from build123d import *

# Parameters (mm, degrees)
SKETCH1_R           = 2.75
BOSS_EXTRUDE1_DEPTH = 2


with BuildPart() as part:
    # Sketch1 → Boss-Extrude1 (new body)
    with BuildSketch(Plane(origin=(0, 0, 0), x_dir=(0, 0, -1), z_dir=(1, 0, 0))):
        with BuildLine():
            Line((4, 4), (44, 4))
            Line((44, 4), (44, -21))
            ThreePointArc((44, -21), (48, -25), (52, -21))
            Line((52, -21), (52, 4))
            Line((52, 4), (77, 4))
            ThreePointArc((77, 4), (81, 8), (77, 12))
            Line((77, 12), (4, 12))
            ThreePointArc((4, 12), (0, 8), (4, 4))
        make_face()
        with Locations((4, 8)):
            Circle(SKETCH1_R, mode=Mode.SUBTRACT)
        with Locations((77, 8)):
            Circle(SKETCH1_R, mode=Mode.SUBTRACT)
        with Locations((48, -21)):
            Circle(SKETCH1_R, mode=Mode.SUBTRACT)
    extrude(amount=-BOSS_EXTRUDE1_DEPTH)


solid = part.part
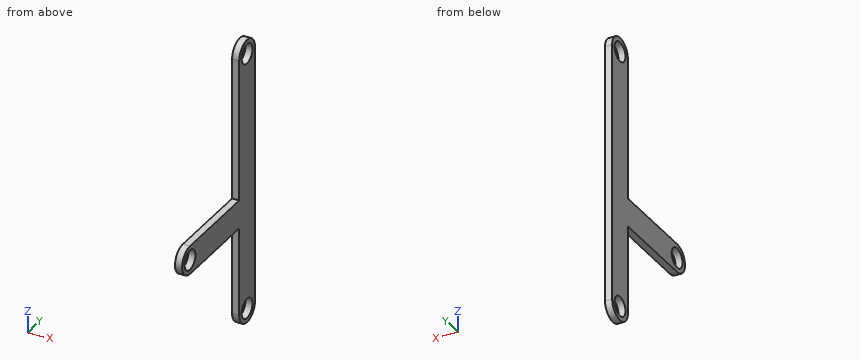
Can you work these out from the model? Positions are in its coordinate system, mm. Give positions to 0.01 mm unless a question says otherwise; leave off trailing zeros. Order: outer loops, then holes, each group sorted by start corner. A loop starts at its lowest first (then second) coordinate and runs counter-clockwise, first axis right, second up. Notation, with made-up numbers: M 39.25,-15 L 65.25,-15 A14 ccw 65.25,7 Z; hole C 4,74.25 d8. An arc over 180 degrees is marked long. Use one line per item in the form item = value. Start each with the question number.
Item 1: Will these pins go through, and if not, where does the flat tip stop? pin 1 Ø9 at (y, z) = (-21, -48) entering from -X; pin 2 Ø1 at (x, z) = (-1, -28) entering from -Y; pin 3 Ø1 at (x, y) = (-0.5, -5.5) entering from -Z.
Item 2: If I drill on line 1 along Y through (x, z) = (-1.1, -48); line 2 along Y through (x, z) = (-0.55, -4); line 3 along Y through (x, z) = (-0.35, -13), over which ranges is the centre line in solid material (lowest first)?
Item 3: If we section it at B-B (x = -0.65): Write out the boundary of the cut face in (y, z), then the cut area to 3 significant figures.
Item 4: If we section it at C-C (z = -48): Write out the boundary of the cut face in (x, y), then the cut area to 3 significant figures.
Item 5: If we section it at D-D (y = -22): Write out the boundary of the cut face in (x, z), then the cut area to 3 significant figures.
Item 6: If we section it at A-A (y = 8): Write out the boundary of the cut face in (x, z), then the cut area to 3 significant figures.
Outcome:
q1.pin_1 = -2
q1.pin_2 = 4
q1.pin_3 = -52
q2.line_1 = -25 to -23.75, -18.25 to 12
q2.line_2 = 4 to 5.25, 10.75 to 12
q2.line_3 = 4 to 12
q3.outline = M -21,-52 L 4,-52 L 4,-77 A4 ccw 12,-77 L 12,-4 A4 ccw 4,-4 L 4,-44 L -21,-44 A4 ccw Z; hole C -21,-48 d5.5; hole C 8,-77 d5.5; hole C 8,-4 d5.5
q3.area = 788 mm2
q4.outline = M -2,-25 L 0,-25 L 0,-23.75 L -2,-23.75 Z; M -2,-18.25 L 0,-18.25 L 0,12 L -2,12 Z
q4.area = 63.0 mm2
q5.outline = M -2,-51.87 L 0,-51.87 L 0,-50.56 L -2,-50.56 Z; M -2,-45.44 L 0,-45.44 L 0,-44.13 L -2,-44.13 Z
q5.area = 5.24 mm2
q6.outline = M -2,-81 L 0,-81 L 0,-79.75 L -2,-79.75 Z; M -2,-74.25 L 0,-74.25 L 0,-6.75 L -2,-6.75 Z; M -2,-1.25 L 0,-1.25 L 0,0 L -2,0 Z
q6.area = 140 mm2
